Check sheet for the drawn part. Datum: minimum x, y, z corner. Units: mm. Give positions to 0.01 mm unless a question says otherwise; leave off trailing zeros. Order: outer loops, then holes, each group sorted by start corner. A loop starts at its lowest first (then second) coordinate and runs counter-clockwise, first axis right, second up.
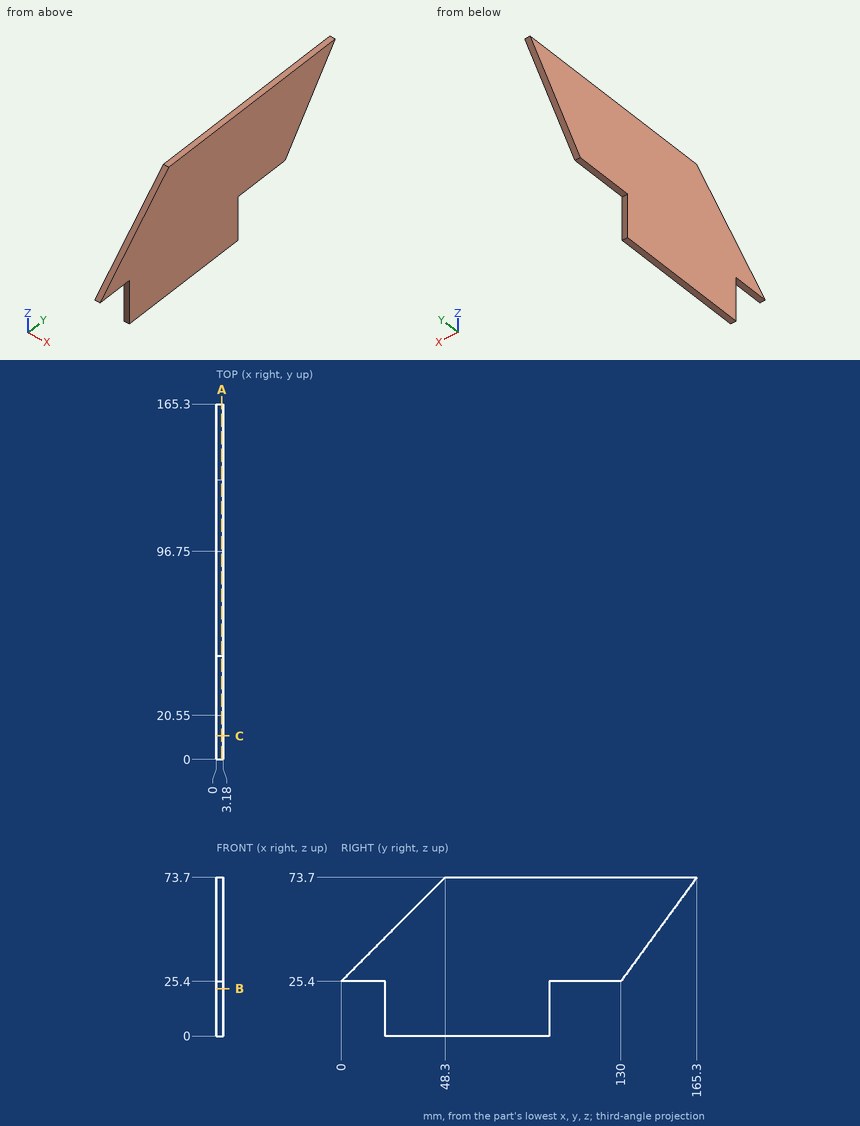
Item 1: Gauge pin test, flat end, axial feed: pin 1 (1 mm diameter, centred on x = 2, y = 109.5, fed in from -Z). Record the tip position at first contact, or that the pin passes through.
Reported:
pin 1: stops at z = 25.4
Item 2: Sectioned sample at C-C (y = 11). Enter the section's corners in (x, z).
Reported:
outline: (0, 25.4) - (3.18, 25.4) - (3.18, 36.4) - (0, 36.4) - close
Item 3: Sectioned sample at A-A (x = 2.55). Enter the section's corners in (y, z).
Reported:
outline: (0, 25.4) - (20.55, 25.4) - (20.55, 0) - (96.75, 0) - (96.75, 25.4) - (130, 25.4) - (165.3, 73.7) - (48.3, 73.7) - close
Item 4: Scan lines: L1, parallel to Y at x = 0.3, z = 13; L2, parallel to Z at x = 2, y = 130; L3, parallel to Y at x = 2.2, z = 56.5. Record each from-to range of solid material in increasing order.
Reported:
L1: y = 20.55 to 96.75
L2: z = 25.4 to 73.7
L3: y = 31.1 to 152.73
Item 5: Sectioned sample at B-B (z = 22). Enter the section's corners in (x, y).
Reported:
outline: (0, 20.55) - (3.18, 20.55) - (3.18, 96.75) - (0, 96.75) - close
